Source: CAD feature listing. Evaluate the final solid. Frame: model axes, mm. A direction names the side the tool comes from. Give positions to 0.01 mm unless a question says otherwise; leave off trailing zeros. Loops run counter-clockwise (first coordinate to the right, second up) from the corner with the lowest first, then second, coordinate; pieces in that order, holes last. Notation, with made-up numbers: (-15, -36.5) - (-1, -36.5) arc R17 cw to (-1, -27.5) - close; hole circle Ø4 at (48, -23). An arc over 180 degrees is marked (long way). Write each question's results on one line, items separated by ' | '. Start each with the question number.
(1) Contact query for flat-ended pins moving along their axis: pin 1 (13 mm diameter, centred on x = 28.28, y = 28.28, fed in from +Z); pin 2 (3 mm diameter, centred on x = 14, z = 1.5, fed in from +Y); pin 3 (1.5 mm diameter, centred on y = -36, z = 2, fed in from +X); pin 4 (1.5 mm diameter, centred on x = 17.5, z = 2.5, fed in from +Y). Output: stop coordinate, or through.
(2) Reachability of faces 4 (the cylindrical face through (47.7, 0.07, 2.47)), 5 (the flat face through (-43.848, 16.054, 2.535)) from +Z, -Z, +X, -X, +Y, -Y: full face, straight path, thin tool, end or side. Return the list, or none.
(3) Cut plane A-A on y = 0. Give the number of separate pieces and of enclosed holes in the cut face, then the cut area to 3 significant figures.
(4) Cut plane B-B on x = 0. Return the cut outline in (y, z), then the cut area to 3 significant figures.
(5) Material intervals for line 1 along Y through (x, z) = (0, 2.45); line 2 along Y through (x, z) = (-3, 2.3); line 3 along Y through (x, z) = (-27, 1.8), sorted ascending. Write a range as [from, to].
(6) Cut plane D-D on x = 46. Return the cut outline in (y, z).
(7) Pull-direction query (X, two-part tool) for faces 1 (the cylindrical face through (35.741, -34.966, 2.465)), 2 (the cylindrical face through (4.864, -38.468, 2.535)), 3 (the flat face through (10, 1, 0)); classes: pulls with the +X half, pulls with the -X half, needs draft (parallel to the pull), parting line crosses it, or undercut.
from build123d import *

# Parameters (mm, degrees)
SKETCH1_R                    = 50
BOSS_EXTRUDE1_DEPTH          = 5
F_15_0_15_DIAMETER_HOLE1_D   = 15
F_10_2_10_2_DIAMETER_HOLE1_D = 10.2
M3_CLEARANCE_HOLE1_D         = 3.4
SKETCH9_R                    = 14.6
SKETCH9_R_2                  = 1.5
CUT_EXTRUDE1_DEPTH           = 10
SKETCH10_R                   = 1.65
CUT_EXTRUDE2_DEPTH           = 5
SKETCH11_R                   = 4
CUT_EXTRUDE3_DEPTH           = 10
FILLET1_R                    = 1


with BuildPart() as part:
    # Sketch1 → Boss-Extrude1 (new body)
    with BuildSketch(Plane.XY):
        Circle(SKETCH1_R)
    extrude(amount=BOSS_EXTRUDE1_DEPTH)

    # Ø15.0 (15) Diameter Hole1 (through all)
    with Locations(Plane(origin=(0, 0, 0), x_dir=(-1, 0, 0), z_dir=(0, 0, -1))):
        with Locations((0, 0)):
            Hole(F_15_0_15_DIAMETER_HOLE1_D / 2)

    # Ø10.2 (10.2) Diameter Hole1 (through all)
    with Locations(Plane(origin=(0, 0, 0), x_dir=(-1, 0, 0), z_dir=(0, 0, -1))):
        with Locations((37, 0), (-37, 0), (0, -40)):
            Hole(F_10_2_10_2_DIAMETER_HOLE1_D / 2)

    # M3 Clearance Hole1 (through all)
    with Locations(Plane.XY.offset(5)):
        with Locations((46, 0), (28, 0), (9, -40), (-9, -40), (-46, 0), (-28, 0)):
            Hole(M3_CLEARANCE_HOLE1_D / 2)

    # Sketch9 → Cut-Extrude1 (cut)
    with BuildSketch(Plane.XY.offset(5)):
        with Locations((24.04163056, -24.04163056)):
            Circle(SKETCH9_R)
        with Locations((10.606601718, -10.606601718)):
            Circle(SKETCH9_R_2)
        with Locations((-24.04163056, -24.04163056)):
            Circle(SKETCH9_R)
        with Locations((-10.606601718, -10.606601718)):
            Circle(SKETCH9_R_2)
        with Locations((0, 34)):
            Circle(SKETCH9_R)
        with Locations((0, 15)):
            Circle(SKETCH9_R_2)
    extrude(amount=-CUT_EXTRUDE1_DEPTH, mode=Mode.SUBTRACT)

    # Sketch10 → Cut-Extrude2 (cut)
    with BuildSketch(Plane.XY.offset(5)):
        with Locations((-20.17442319, 27.477446333)):
            Circle(SKETCH10_R)
        with Locations((-29.722400231, 17.23849451)):
            Circle(SKETCH10_R)
        with BuildLine():
            Line((-27.274837591, 48.455628221), (-18.498593172, 40.2716479))
            ThreePointArc((-18.498593172, 40.2716479), (-17.546415771, 38.182285285), (-18.350527147, 36.031591715))
            Line((-18.350527147, 36.031591715), (-38.128479589, 14.822334368))
            ThreePointArc((-38.128479589, 14.822334368), (-40.217842204, 13.870156967), (-42.368535774, 14.674268343))
            Line((-42.368535774, 14.674268343), (-51.144780194, 22.858248664))
            Line((-51.144780194, 22.858248664), (-27.274837591, 48.455628221))
        make_face()
    extrude(amount=-CUT_EXTRUDE2_DEPTH, mode=Mode.SUBTRACT)

    # Sketch11 → Cut-Extrude3 (cut)
    with BuildSketch(Plane.XY.offset(5)):
        with Locations((28.284271247, 28.284271247)):
            Circle(SKETCH11_R)
    extrude(amount=-CUT_EXTRUDE3_DEPTH, mode=Mode.SUBTRACT)

    # Fillet1
    fillet1_edges = [part.edges().sort_by_distance(p)[0] for p in [
        (-46.456878561, 18.486709669, 2.5),
        (-22.949421323, 44.422112297, 2.5),
    ]]
    fillet(fillet1_edges, radius=FILLET1_R)


solid = part.part
Ans:
1) pin 1: z = 5 | pin 2: y = 48.41 | pin 3: x = 35.46 | pin 4: y = 47.11
2) face 4: +Z, -Z | face 5: +Z, -Z, +Y
3) separate pieces: 8 | enclosed holes: 0 | area: 255 mm^2
4) outline: (-50, 0) - (-45.1, 0) - (-45.1, 5) - (-50, 5) - close; (-34.9, 0) - (-7.5, 0) - (-7.5, 5) - (-34.9, 5) - close; (7.5, 0) - (13.5, 0) - (13.5, 5) - (7.5, 5) - close; (16.5, 0) - (19.4, 0) - (19.4, 5) - (16.5, 5) - close; (48.6, 0) - (50, 0) - (50, 5) - (48.6, 5) - close | area: 213 mm^2
5) line 1: [-50, -45.1], [-34.9, -7.5], [7.5, 13.5], [16.5, 19.4], [48.6, 50] | line 2: [-49.91, -44.12], [-35.88, -6.87], [6.87, 19.71], [48.29, 49.91] | line 3: [-42.08, -38.34], [-9.74, -1.37], [1.37, 26.76]
6) outline: (-19.6, 0) - (-1.7, 0) - (-1.7, 5) - (-19.6, 5) - close; (1.7, 0) - (19.6, 0) - (19.6, 5) - (1.7, 5) - close
7) face 1: parting line crosses it | face 2: undercut | face 3: needs draft
